```python
from build123d import *
from build123d.topology import SkipClean

# Parameters (mm, degrees)
SKETCH1_R           = 29
SKETCH1_R_2         = 2.0000000000000013
SKETCH1_R_3         = 2.00000000000017
SKETCH1_R_4         = 2.0000000000003304
BOSS_EXTRUDE1_DEPTH = 3
BOSS_EXTRUDE2_DEPTH = 35
FILLET1_R           = 14
CHAMFER1_SIZE       = 3


# Some blends are built 0.0001 mm under size
with BuildPart() as part:
    # Sketch1 → Boss-Extrude1 (new body)
    with BuildSketch(Plane(origin=(0, 0, 0), x_dir=(1, 0, 0), z_dir=(0, 1, 0))):
        with BuildLine():
            ThreePointArc((-12.355312859352809, 29.51857456157921), (-27.71281292110204, 15.999999999999998), (-31.741491883509095, -4.0592724728855325))
            ThreePointArc((-31.741491883509095, -4.0592724728855325), (-32.309645144827726, -8.871468590740253), (-35.073430755727436, -12.851609128714605))
            ThreePointArc((-35.073430755727436, -12.851609128714605), (-36.427364069331304, -21.031348451296957), (-28.666535362838538, -23.948677467977124))
            ThreePointArc((-28.666535362838538, -23.948677467977124), (-23.83773974087064, -23.54523918731126), (-19.38617902415628, -25.4593020886937))
            ThreePointArc((-19.38617902415628, -25.4593020886937), (1.617e-14, -32.00000000000001), (19.386179024156295, -25.45930208869368))
            ThreePointArc((19.386179024156295, -25.45930208869368), (23.837739740870653, -23.54523918731124), (28.666535362838555, -23.948677467977113))
            ThreePointArc((28.666535362838555, -23.948677467977113), (36.427364069331325, -21.031348451296928), (35.07343075572746, -12.851609128714571))
            ThreePointArc((35.07343075572746, -12.851609128714571), (32.30964514482773, -8.87146859074023), (31.741491883509102, -4.059272472885512))
            ThreePointArc((31.741491883509102, -4.059272472885512), (27.712812921102042, 16.000000000000007), (12.355312859352809, 29.518574561579204))
            ThreePointArc((12.355312859352809, 29.518574561579204), (8.47190540395708, 32.41670777805148), (6.4068953928889005, 36.8002865966917))
            ThreePointArc((6.4068953928889005, 36.8002865966917), (4.75e-15, 42.06269690259387), (-6.406895392888902, 36.800286596691706))
            ThreePointArc((-6.406895392888902, 36.800286596691706), (-8.471905403957084, 32.41670777805149), (-12.355312859352809, 29.51857456157921))
        make_face()
        with Locations(Location((0, 0, 0), (0, 0, 270))):
            Circle(SKETCH1_R, mode=Mode.SUBTRACT)
        with Locations(Location((0, 35.53134845129693, 0), (0, 0, 270))):
            Circle(SKETCH1_R_2, mode=Mode.SUBTRACT)
        with Locations(Location((30.771050389540026, -17.76567422564846, 0), (0, 0, 270))):
            Circle(SKETCH1_R_3, mode=Mode.SUBTRACT)
        with Locations(Location((-30.771050389540008, -17.765674225648485, 0), (0, 0, 270))):
            Circle(SKETCH1_R_4, mode=Mode.SUBTRACT)
    extrude(amount=BOSS_EXTRUDE1_DEPTH)

    # Sketch2 → Boss-Extrude2 (add)
    with SkipClean():  # the faces are left unmerged after this step: merging them gives an invalid solid
        with BuildSketch(Plane(origin=(0, 3, 0), x_dir=(1, 0, 0), z_dir=(0, 1, 0))):
            with BuildLine():
                Line((-15.556616883168559, 27.964113988294258), (-14.098184050372366, 25.34247830189322))
                ThreePointArc((-14.098184050372366, 25.34247830189322), (-0.11887275101926295, 28.999756365686377), (13.88995133460985, 25.457204322593487))
                Line((13.88995133460985, 25.457204322593487), (15.326842851982352, 28.09070821803249))
                ThreePointArc((15.326842851982352, 28.09070821803249), (-0.13116993215917874, 31.99973116213475), (-15.556616883168559, 27.964113988294258))
            make_face()
            with BuildLine():
                Line((-28.991561320001907, -0.699551448195039), (-31.990688353103597, -0.7719188393875828))
                ThreePointArc((-31.990688353103597, -0.7719188393875828), (-27.646995134601628, -16.1134620745299), (-16.439324666602317, -27.454482411913002))
                Line((-16.439324666602317, -27.454482411913002), (-14.898137979109256, -24.88062468579768))
                ThreePointArc((-14.898137979109256, -24.88062468579768), (-25.055089340734252, -14.602825005043623), (-28.991561320001907, -0.699551448195039))
            make_face()
            with BuildLine():
                Line((31.995941549770887, -0.5096315763812559), (28.996322029481636, -0.46185361609554243))
                ThreePointArc((28.996322029481636, -0.46185361609554243), (25.173962091753527, -14.396931360642762), (15.101609985392061, -24.757652874398442))
                Line((15.101609985392061, -24.757652874398442), (16.663845501121262, -27.318789378644897))
                ThreePointArc((16.663845501121262, -27.318789378644897), (27.778165066760824, -15.88626908760484), (31.995941549770887, -0.5096315763812559))
            make_face()
        extrude(amount=BOSS_EXTRUDE2_DEPTH)

    # Fillet1
    # the kernel refuses this fillet: 14 mm, written as the material it adds along each edge
    with BuildSketch(Plane(origin=(-32.57166659913419, 3, -58.5498636629911), x_dir=(0, 1, 0), z_dir=(0.486144277599018, 0, 0.8738785621341955))) as fillet1_piece_1_section:
        with BuildLine():
            CenterArc((FILLET1_R, FILLET1_R), FILLET1_R, 180.00000000000003, 90)
            Line((0, FILLET1_R), (0, 0))
            Line((0, 0), (FILLET1_R, 0))
        make_face()
    fillet1_piece_1 = extrude(amount=72.99999999999824, mode=Mode.PRIVATE)
    fillet1_piece_1 = fillet1_piece_1 & Plane(origin=(1.377e-14, 6.144013210194413, -4.086e-14), x_dir=(0.4789638391244486, 0, -0.877834631813515), z_dir=(0, -1, 0)) * Cylinder(31.99999999999996, 202, mode=Mode.PRIVATE)
    fillet1_piece_1 = fillet1_piece_1 - Plane(origin=(0, 6.144013210194413, 0), x_dir=(-1.8e-16, 0, 1), z_dir=(0, -1, 0)) * Cylinder(29, 202, mode=Mode.PRIVATE)
    add(fillet1_piece_1)
    with BuildSketch(Plane(origin=(-2.8737830347458213, 3, 5.267007790879544), x_dir=(0.8778346318135153, 0, 0.4789638391244479), z_dir=(0.4789638391244479, 0, -0.8778346318135153))) as fillet1_piece_2_section:
        with BuildLine():
            CenterArc((FILLET1_R, -FILLET1_R), FILLET1_R, 90, 90)
            Line((-2.37e-15, -FILLET1_R), (0, 0))
            Line((0, 0), (FILLET1_R, 0))
        make_face()
    fillet1_piece_2 = extrude(amount=72.99999999999824, mode=Mode.PRIVATE)
    fillet1_piece_2 = fillet1_piece_2 & Plane(origin=(5.151e-14, 6.1440139073006, -2.487e-14), x_dir=(0.9919216213596592, 0, 0.12685226477767322), z_dir=(0, -1, 0)) * Cylinder(31.999999999999954, 202, mode=Mode.PRIVATE)
    fillet1_piece_2 = fillet1_piece_2 - Plane(origin=(0, 6.1440139073006, 0), x_dir=(-1.8e-16, 0, 1), z_dir=(0, -1, 0)) * Cylinder(29, 202, mode=Mode.PRIVATE)
    add(fillet1_piece_2)
    with BuildSketch(Plane(origin=(66.99150261983281, 3, 1.0670411130482422), x_dir=(0.015925986761913882, 0, -0.9998731734303402), z_dir=(-0.9998731734303404, 0, -0.015925986761913886))) as fillet1_piece_3_section:
        with BuildLine():
            CenterArc((FILLET1_R, -FILLET1_R), FILLET1_R, 90, 90)
            Line((0, -FILLET1_R), (0, 0))
            Line((0, 0), (FILLET1_R, 0))
        make_face()
    fillet1_piece_3 = extrude(amount=72.99999999999828, mode=Mode.PRIVATE)
    fillet1_piece_3 = fillet1_piece_3 & Plane(origin=(5.151e-14, 6.144014691753946, -2.487e-14), x_dir=(0.9919216213596592, 0, 0.12685226477767322), z_dir=(0, -1, 0)) * Cylinder(31.999999999999954, 202, mode=Mode.PRIVATE)
    fillet1_piece_3 = fillet1_piece_3 - Plane(origin=(0, 6.144014691753946, 0), x_dir=(-1.8e-16, 0, 1), z_dir=(0, -1, 0)) * Cylinder(29, 202, mode=Mode.PRIVATE)
    add(fillet1_piece_3)
    with BuildSketch(Plane(origin=(-3.124471031459313, 3, -5.122273008494407), x_dir=(0, 1, 0), z_dir=(0.5207451719100392, 0, 0.8537121680826528))) as fillet1_piece_4_section:
        with BuildLine():
            CenterArc((FILLET1_R, FILLET1_R), FILLET1_R, 180, 90)
            Line((0, FILLET1_R), (0, 0))
            Line((0, 0), (FILLET1_R, 0))
        make_face()
    fillet1_piece_4 = extrude(amount=72.99999999999824, mode=Mode.PRIVATE)
    fillet1_piece_4 = fillet1_piece_4 & Plane(origin=(1.066e-14, 6.144012485408136, 2.132e-14), x_dir=(0.5207451719100394, 0, 0.8537121680826528), z_dir=(0, -1, 0)) * Cylinder(31.999999999999986, 202, mode=Mode.PRIVATE)
    fillet1_piece_4 = fillet1_piece_4 - Plane(origin=(0, 6.144012485408136, 0), x_dir=(-1.8e-16, 0, 1), z_dir=(0, -1, 0)) * Cylinder(29, 202, mode=Mode.PRIVATE)
    add(fillet1_piece_4)
    with BuildSketch(Plane(origin=(5.998254066205156, 3, -0.1447347823851374), x_dir=(-0.024122463730862184, 0, -0.9997090110344876), z_dir=(-0.9997090110344876, 0, 0.024122463730862184))) as fillet1_piece_5_section:
        with BuildLine():
            CenterArc((FILLET1_R, -FILLET1_R), FILLET1_R, 90, 90)
            Line((-1.64e-15, -FILLET1_R), (0, 0))
            Line((0, 0), (FILLET1_R, 0))
        make_face()
    fillet1_piece_5 = extrude(amount=72.99999999999821, mode=Mode.PRIVATE)
    fillet1_piece_5 = fillet1_piece_5 & Plane(origin=(-8.88e-15, 6.144013907117808, -9.33e-15), x_dir=(-0.3861035268547751, 0, -0.9224554550493503), z_dir=(0, -1, 0)) * Cylinder(31.999999999999986, 202, mode=Mode.PRIVATE)
    fillet1_piece_5 = fillet1_piece_5 - Plane(origin=(0, 6.144013907117808, 0), x_dir=(-1.8e-16, 0, 1), z_dir=(0, -1, 0)) * Cylinder(29, 202, mode=Mode.PRIVATE)
    add(fillet1_piece_5)
    with BuildSketch(Plane(origin=(-34.41983602069866, 3, 57.48282254994282), x_dir=(0.8579525753722805, 0, 0.513728895831324), z_dir=(0.513728895831324, 0, -0.8579525753722805))) as fillet1_piece_6_section:
        with BuildLine():
            CenterArc((FILLET1_R, -FILLET1_R), FILLET1_R, 90, 90)
            Line((3.65e-15, -FILLET1_R), (0, 0))
            Line((0, 0), (FILLET1_R, 0))
        make_face()
    fillet1_piece_6 = extrude(amount=72.99999999999822, mode=Mode.PRIVATE)
    fillet1_piece_6 = fillet1_piece_6 & Plane(origin=(-7.99e-15, 6.144014691708705, 8.88e-15), x_dir=(-0.6058180945048837, 0, 0.795603190271678), z_dir=(0, -1, 0)) * Cylinder(31.999999999999996, 202, mode=Mode.PRIVATE)
    fillet1_piece_6 = fillet1_piece_6 - Plane(origin=(0, 6.144014691708705, 0), x_dir=(-1.8e-16, 0, 1), z_dir=(0, -1, 0)) * Cylinder(29, 202, mode=Mode.PRIVATE)
    add(fillet1_piece_6)

    # Chamfer1
    chamfer1_edges = [part.edges().sort_by_distance(p)[0] for p in [
        (-0.1188727510192642, 38, -28.999756365686377),
        (25.173962091753527, 38, 14.39693136064276),
        (-25.055089340734256, 38, 14.60282500504362),
    ]]
    chamfer(chamfer1_edges, length=CHAMFER1_SIZE - 0.0001)  # a hair under: the kernel refuses the full size


solid = part.part
```
Work out the finished part from the listing and answer in its coordinate system (mm). A direction names the side the tool comes from. Round coordinates to 2 decimals unless told otherwise and drop trailing zeros. Write each loop counter-clockwise with the first axis right and the second up, starting at its lowest first coordinate (ties: lowest second). Pieces come first, ordered by that corner, then holes. Notation, with made-up numbers: (88, 22.5) - (112, 22.5) arc R32 ccw to (112, 53.5) - close; hole circle Ø3 at (43, 36). An arc over 180 degrees is marked (long way). Return JSON: item names as keys, results as strings. Group by question number.
Q1. Find the intervals of material crossed by L1, parallel to X at y = 2, z = 0; L2, parallel to X at y = 9, z = 4.5; L3, parallel to Y at x = 28, z = -13, in increasing order.
Q2. The mould has two halves that part along Z. Classify faces 1 (the cylindrical face through (11.708, 6.992, 27.279)), 2 (the cylindrical face through (-32.286, 1.479, 8.807)), 3 (the cylindrical face through (0.13, 1.48, -42.06)): released by +Z, released by -Z, zero draft, split by the parting line, or undercut.
Q3. The part is cut by section C-C on y = 9. Write down the section's boundary in (x, z), then the cut area to 3 significant figures.
Q4. For faces 4 (the cylindrical face through (-18.01, 6.99, -23.71)), 5 (the flat face through (0, 3, 31)), 6 (the flat face through (-33, 3, 18)), determine the directions among +Z, -Z, +X, -X, +Y, -Y from which every point of the face is accessible in a straight line to the end or side of a thin tool.
Q5. Each of these flat-tipped pins is pushed along its axis until it touches: pin 1 Ø2.5 at (x, z) = (-0.5, 31) entering from +Y; pin 2 Ø5 at (x, y) = (-8.5, 13.5) entering from +Z; pin 3 Ø6 at (x, y) = (11.5, 28.5) entering from +Z. Where does it stop, or does it pass through?
Q6. The part is cut by section B-B on y = 24.5. Write down the section's boundary in (x, z).
Q7. The part is cut by section A-A on x = 0. Count the separate pieces of the cut face and the enclosed holes in it, then the cut area to 3 significant figures.
Solved:
{
 "1": {"L1": "-32 to -29, 29 to 32", "L2": "-31.68 to -28.65, 28.65 to 31.68", "L3": "0 to 3.01"},
 "2": {"face 1": "released by +Z", "face 2": "undercut", "face 3": "released by -Z"},
 "3": {"outline": "(-31.95, -1.74) - (-28.94, -1.81) arc R29 cw to (-12.69, 26.08) - (-14.23, 28.66) arc R32 ccw to start; (-17.7, -26.66) arc R32 ccw to (17.48, -26.8) - (16.04, -24.16) arc R29 cw to (-16.24, -24.03) - close; (12.9, 25.97) arc R29 cw to (28.93, -2.05) - (31.94, -2) arc R32 ccw to (14.47, 28.54) - close", "area": "322 mm²"},
 "4": {"face 4": "-X, +Y", "face 5": "+Z, +Y", "face 6": "+Z, -X, +Y"},
 "5": {"pin 1": "y = 3", "pin 2": "z = -26.83", "pin 3": "z = -25.46"},
 "6": {"outline": "(-31.99, 0.77) - (-28.99, 0.7) arc R29 cw to (-14.9, 24.88) - (-16.44, 27.45) arc R32 ccw to start; (-15.56, -27.96) arc R32 ccw to (15.33, -28.09) - (13.89, -25.46) arc R29 cw to (-14.1, -25.34) - close; (15.1, 24.76) arc R29 cw to (29, 0.46) - (32, 0.51) arc R32 ccw to (16.66, 27.32) - close"},
 "7": {"separate pieces": "3", "enclosed holes": "0", "area": "137 mm²"}
}
